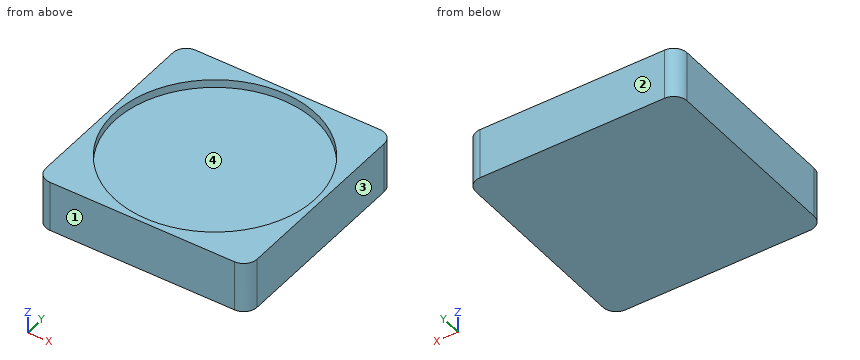
```python
from build123d import *

# Parameters (mm, degrees)
SKETCH1_W           = 158
SKETCH1_H           = 158
BOSS_EXTRUDE1_DEPTH = 38
SKETCH2_R           = 75
CUT_EXTRUDE1_DEPTH  = 6
FILLET1_R           = 10


with BuildPart() as part:
    # Sketch1 → Boss-Extrude1 (new body)
    with BuildSketch(Plane.XY):
        with Locations((79, -79)):
            Rectangle(SKETCH1_W, SKETCH1_H)
    extrude(amount=BOSS_EXTRUDE1_DEPTH)

    # Sketch2 → Cut-Extrude1 (cut)
    with BuildSketch(Plane.XY.offset(38)):
        with Locations((79, -79)):
            Circle(SKETCH2_R)
    extrude(amount=-CUT_EXTRUDE1_DEPTH, mode=Mode.SUBTRACT)

    # Fillet1
    fillet1_edges = [part.edges().sort_by_distance(p)[0] for p in [
        (0, 0, 19),
        (158, 0, 19),
        (158, -158, 19),
        (0, -158, 19),
    ]]
    fillet(fillet1_edges, radius=FILLET1_R)


solid = part.part
```
Geometry: final body of the model. Coordinates: model frame, mm. Face numbers are marked on the shaded views. Round coordinates to 2 decimals unless told otherwise and drop trailing zeros. Write each loop counter-clockwise with the first axis right and the second up, starting at its lowest first coordinate (ties: lowest second). Pieces come first, ordered by that corner, then holes.
Item 1: Section query A-A (y = -34). Return loops of the section in (x, z).
Item 2: Material intervals for L1, parallel to Y at x = 79, z = 35; L2, parallel to Z at x = 42.5, y = -19.5; L3, parallel to Y at x = 33.5, z = 35.5, sorted ascending.
Item 3: Mould query, pull axis Y, two halves, no side actions, for the marked faces 1, 2, 3 and 4. Classes: +Y half, -Y half, draft (parallel to the pull), parting line (faces both ways), or undercut.
Item 4: Section query B-B (x = 79). Return loops of the section in (y, z).
Item 5: Pin query (flat end, axial travel): P1, Ø1, axis at x = 107, y = -53, coming from the +Z side. Return the tip coordinate at first contact, or that it passes through.
Completed:
1. outline: (0, 0) - (158, 0) - (158, 38) - (139, 38) - (139, 32) - (19, 32) - (19, 38) - (0, 38) - close
2. L1: y = -158 to -154, -4 to 0
2. L2: z = 0 to 32
2. L3: y = -158 to -138.62, -19.38 to 0
3. face 1: -Y half
3. face 2: +Y half
3. face 3: draft
3. face 4: undercut
4. outline: (-158, 0) - (0, 0) - (0, 38) - (-4, 38) - (-4, 32) - (-154, 32) - (-154, 38) - (-158, 38) - close
5. P1: stops at z = 32
